from build123d import *

# Parameters (mm, degrees)
SKETCH1_W           = 30.48
SKETCH1_H           = 34.544
BOSS_EXTRUDE1_DEPTH = 3.175
SKETCH2_W           = 6.35
SKETCH2_H           = 6.35
BOSS_EXTRUDE2_DEPTH = 6.35
SKETCH5_W           = 10.16
SKETCH5_H           = 6.35
BOSS_EXTRUDE4_DEPTH = 6.35
CAVITY1_START       = 1.778
CAVITY1_OUTLINE_W   = 10.16
CAVITY1_OUTLINE_H   = 6.35
CAVITY1_DEPTH       = 6.35


# Read off the part's stored shape, not the designer's step: Cavity1
with BuildPart() as part:
    # Sketch1 → Boss-Extrude1 (new, symmetric)
    with BuildSketch(Plane.XY):
        Rectangle(SKETCH1_W, SKETCH1_H)
    extrude(amount=BOSS_EXTRUDE1_DEPTH, both=True)

    # Sketch2 → Boss-Extrude2 (add)
    with BuildSketch(Plane.XY.offset(3.175)):
        with Locations((18.415, -7.387912323)):
            Rectangle(SKETCH2_W, SKETCH2_H)
    extrude(amount=-BOSS_EXTRUDE2_DEPTH)

    # Sketch5 → Boss-Extrude4 (add)
    with BuildSketch(Plane.XY.offset(3.175)):
        with Locations((0, -20.447)):
            Rectangle(SKETCH5_W, SKETCH5_H)
    extrude(amount=-BOSS_EXTRUDE4_DEPTH)

    # Cavity1 outline → Cavity1 (cut)
    with BuildSketch(Plane(origin=(0, 0, 0), x_dir=(1, 0, 0), z_dir=(0, 1, 0)).offset(CAVITY1_START)):
        with Locations((0.138449205, 0)):
            Rectangle(CAVITY1_OUTLINE_W, CAVITY1_OUTLINE_H)
    extrude(amount=CAVITY1_DEPTH, mode=Mode.SUBTRACT)


solid = part.part
Geometry: final body of the model. Coordinates: model frame, mm. A direction names the side the tool comes from. Give positions to 0.01 mm unless a question says otherwise; leave off trailing zeros. Loops run counter-clockwise (first coordinate to the right, second up) from the corner with the lowest first, then second, coordinate; pieces in that order, holes last. Notation, with made-up numbers: (31.5, 27) - (69.5, 27) arc R35 cw to (69.5, 59) - close; hole circle Ø2 at (23, 66.5). An arc over 180 degrees is marked (long way). One line per question, with ' | ' between items. Start each with the question number.
(1) Section query D-D on x = -6. Return loops of the section in (y, z) (3 decimals), then the cut area to 3 significant figures.
(2) Section query B-B on y = 7. Return loops of the section in (x, z) (3 decimals).
(3) Reachability of faces 1 (the flat face through (5.08, -20, 0)), 2 (the flat face through (-5.08, -20, 0)), 3 (the flat face through (5.218, 5, 0)), 4 (the flat face through (18, -4.213, 0)) from +Z, -Z, +X, -X, +Y, -Y: full face, straight path, thin tool, end or side. Return the list, or none.
(4) Contact query for flat-ended pins moving along their axis: pin 1 (1.9 mm diameter, centred on y = -14.5, z = 0.5, fed in from +X); pin 2 (3 mm diameter, centred on x = -12.5, z = 1, fed in from -Y). Output: stop coordinate, or through.
(5) Section query A-A on z = 1.5. Return loops of the section in (x, y), then the cut area to 3 significant figures.
(6) Ray query, line 1 (Y direction, x = 0, z = -2.5); line 2 (X direction, y = 2.5, z = 0.25); line 3 (X direction, y = -0.5, z = 0). Return the intervals inside material, ascending. Write a range as from..to.
(7) Section query C-C on x = 0.5. Return loops of the section in (y, z) (3 decimals), then the cut area to 3 significant figures.
(8) Pull-direction query (X, two-part tool) for faces 5 (the flat face through (-15.24, 0, 0)), 6 (the flat face through (0, 8.128, 0)), 7 (the flat face through (-4.942, 5, 0)), 8 (the flat face through (10, -17.272, 0)); classes: released by +X, released by -X, zero draft, split by the parting line, or undercut.
The answers:
1) outline: (-17.272, -3.175) - (17.272, -3.175) - (17.272, 3.175) - (-17.272, 3.175) - close | area: 219 mm2
2) outline: (-15.24, -3.175) - (-4.942, -3.175) - (-4.942, 3.175) - (-15.24, 3.175) - close; (5.218, -3.175) - (15.24, -3.175) - (15.24, 3.175) - (5.218, 3.175) - close
3) face 1: +Z, -Z, +X, -Y | face 2: +Z, -Z, -X, -Y | face 3: +Z, -Z | face 4: +Z, -Z, +X, +Y
4) pin 1: x = 15.24 | pin 2: y = -17.27
5) outline: (-15.24, -17.27) - (-5.08, -17.27) - (-5.08, -23.62) - (5.08, -23.62) - (5.08, -17.27) - (15.24, -17.27) - (15.24, -10.56) - (21.59, -10.56) - (21.59, -4.21) - (15.24, -4.21) - (15.24, 17.27) - (-15.24, 17.27) - close; hole (-4.94, 1.78) - (5.22, 1.78) - (5.22, 8.13) - (-4.94, 8.13) - close | area: 1,090 mm2
6) line 1: -23.62..1.78, 8.13..17.27 | line 2: -15.24..-4.94, 5.22..15.24 | line 3: -15.24..15.24
7) outline: (-23.622, -3.175) - (1.778, -3.175) - (1.778, 3.175) - (-23.622, 3.175) - close; (8.128, -3.175) - (17.272, -3.175) - (17.272, 3.175) - (8.128, 3.175) - close | area: 219 mm2
8) face 5: released by -X | face 6: undercut | face 7: undercut | face 8: zero draft
